Input: dimensioned drawing with shaded views. Units: mm. Origin: part minimum x, y, z. Round coordinates to 2 decimals unless told otherwise and drop trailing zeros. Write each loop counter-clockwise with the first axis right and the second up, starting at its lowest first coordinate (ties: lowest second). Pieces come first, ordered by that corner, then holes. Notation, with made-up numbers: (62, 37.25) -> (113, 37.25) arc R14 ccw to (113, 64.25) -> close; hole circle Ø5 at (0.25, -6). An arc over 180 degrees is marked (long way). One line per item, written item: value. Start each with the question number.
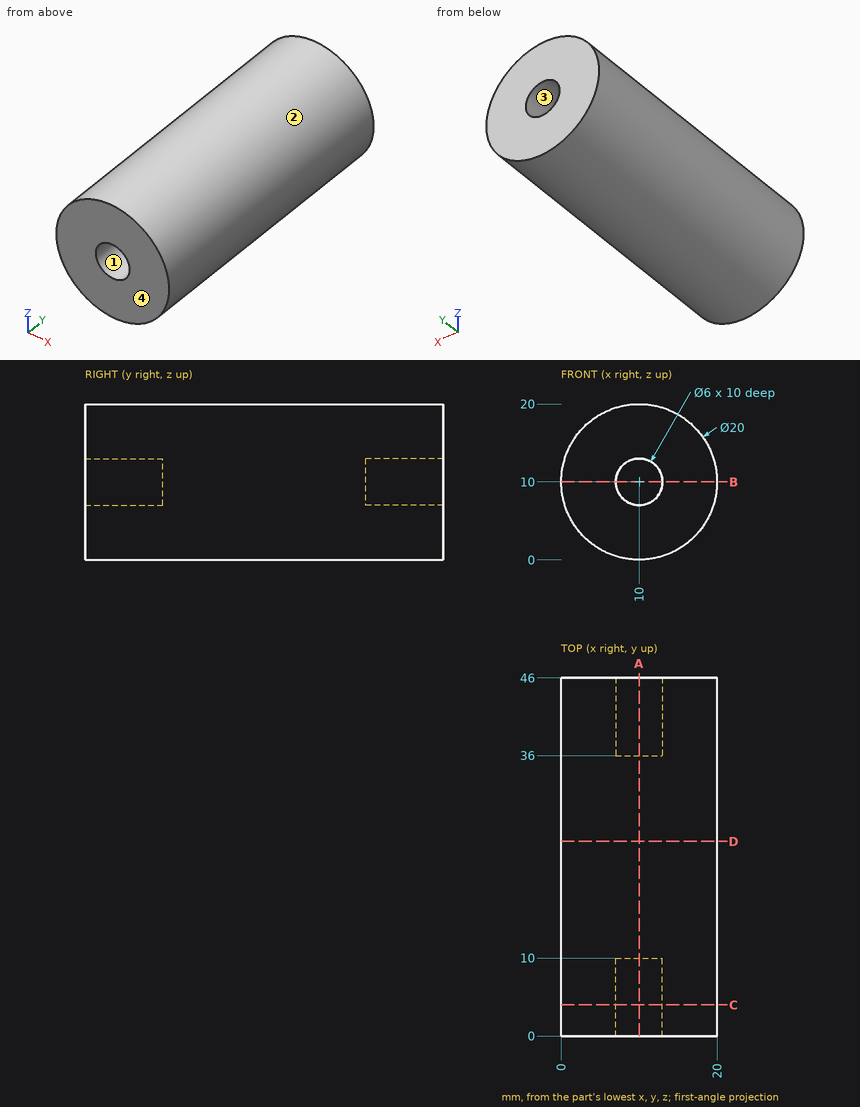
(1) Section query B-B (z = 10). Output: boundary loops of the cut face in (x, y), and give its area (3 significant figures).
(2) Section query A-A (x = 10). Output: boundary loops of the cut face in (y, z).
(3) Pin query (flat end, axial travel): pin 1 (6 mm diameter, centred on y = 39.5, z = 12.5, fed in from +X); pin 2 (3.5 mm diameter, centred on x = 10, z = 10, fed in from +Y); pin 3 (2 mm diameter, centred on x = 13, y = 34.5, fed in from +Z); pin 4 (1.5 mm diameter, centred on x = 13, y = 17.5, fed in from +Z). Return the tip coordinate at first contact, or that it passes through.
(4) Pull-direction query (X, two-part tool) for the marked faces 1, 2, 3 and 4; classes: pulls with the +X half, pulls with the -X half, needs draft (parallel to the pull), parting line crosses it, or undercut.
(5) Line query: probe 1 along Z at (x, y) = (10, 41); probe 2 along Y at (x, z) = (12, 9); probe 3 along X at (y, z) = (3, 12). Output: solid intervals per line, ascending.
(6) Section query D-D (y = 25). Output: boundary loops of the cut face in (x, z), and give its area (3 significant figures).
(7) Section query C-C (y = 4). Output: boundary loops of the cut face in (x, z), and give its area (3 significant figures).
Results list:
1. outline: (0, 0) -> (7, 0) -> (7, 10) -> (13, 10) -> (13, 0) -> (20, 0) -> (20, 46) -> (13, 46) -> (13, 36) -> (7, 36) -> (7, 46) -> (0, 46) -> close
1. area: 800 mm^2
2. outline: (0, 0) -> (46, 0) -> (46, 7) -> (36, 7) -> (36, 13) -> (46, 13) -> (46, 20) -> (0, 20) -> (0, 13) -> (10, 13) -> (10, 7) -> (0, 7) -> close
3. pin 1: stops at x = 20
3. pin 2: stops at y = 36
3. pin 3: stops at z = 19.8
3. pin 4: stops at z = 19.74
4. face 1: undercut
4. face 2: parting line crosses it
4. face 3: undercut
4. face 4: needs draft
5. probe 1: z = 0 to 7, 13 to 20
5. probe 2: y = 10 to 36
5. probe 3: x = 0.2 to 7.76, 12.24 to 19.8
6. outline: circle Ø20 at (10, 10)
6. area: 314 mm^2
7. outline: circle Ø20 at (10, 10); hole circle Ø6 at (10, 10)
7. area: 286 mm^2
